Verification items for the finished model (mm, model axes). Face numbers are marked on the shaded views. A direction names the side the tool comes from. Coordinates: 2 decimals unless noted, no trailing zeros. Loops run counter-clockwise (first coordinate to the right, second up) from the corner with the lowest first, then second, coordinate; pieces in that order, holes last. Notation, with made-up numbers: (23, 63) -> (37, 63) arc R29 ccw to (37, 97) -> close; hole circle Ø9 at (79, 41.25). An arc over 180 degrees is marked (long way). Write item = value, one per line.
Autodesk Inventor part; units mm, degrees
ref_plane "Work Plane2" through (-20, 0, -10) normal (0, 0, 1) x (1, 0, 0)
ref_plane "Work Plane3" through (0, 8, 0) normal (0, 1, 0) x (1, 0, 0)
ref_plane "YZ Plane" through (0, 0, 0) normal (1, 0, 0) x (0, 1, 0)
sketch "Sketch1" plane through (0, 0, 0) normal (0, 1, 0) x (-1, 0, 0)
  line L0 (0, 0) -> (20, 0)
  line L1 (20, 0) -> (20, -20)
  line L2 (20, -20) -> (0, -20)
  line L3 (0, -20) -> (0, 0)
  dimension "d0" = 20
  dimension "d1" = 20
extrude "Extrusion1" add sketch "Sketch1" along normal blind 10
sketch "Sketch4" plane through (0, 10, 0) normal (0, 1, 0) x (1, 0, 0)
  line L0 (0, 20) -> (-20, 20)
  line L1 (-20, 20) -> (-20, 0)
  line L2 (-20, 0) -> (0, 0)
  line L3 (0, 0) -> (0, 20)
  line L4 (0, 20) -> (-20, 20)
  line L5 (-20, 20) -> (0, 0)
  line L6 (-10.1768, 10.1768) -> (-7.7019, 12.6517)
  line L7 (-7.7019, 12.6517) -> (-5.227, 10.1768)
  line L8 (-5.227, 10.1768) -> (-7.7019, 7.7019)
  line L9 (-7.7019, 7.7019) -> (-10.1768, 10.1768)
  line L10 (-10.1768, 10.1768) -> (-12.6517, 7.7019)
  line L11 (-12.6517, 7.7019) -> (-15.1265, 10.1768)
  line L12 (-15.1265, 10.1768) -> (-12.6517, 12.6517)
  line L13 (-12.6517, 12.6517) -> (-10.1768, 10.1768)
  line L14 (-12.6517, 12.6517) -> (-10.1768, 15.1265)
  line L15 (-10.1768, 15.1265) -> (-7.7019, 12.6517)
  line L16 (-7.7019, 12.6517) -> (-10.1768, 10.1768)
  line L17 (-10.1768, 10.1768) -> (-12.6517, 12.6517)
  line L18 (-12.6517, 7.7019) -> (-10.1768, 10.1768)
  line L19 (-10.1768, 10.1768) -> (-7.7019, 7.7019)
  line L20 (-7.7019, 7.7019) -> (-10.1768, 5.227)
  line L21 (-10.1768, 5.227) -> (-12.6517, 7.7019)
  dimension "d10" = 3.5
  dimension "d11" = 3.5
  dimension "d12" = 3.5
  dimension "d13" = 3.5
extrude "Extrusion3" cut sketch "Sketch4" against normal blind 8 contours L14 L15 L6 L5 | L5 L10 L11 L12 | L20 L21 L10 L5 | L5 L6 L7 L8
sketch "Sketch5" plane through (0, 10, 0) normal (0, 1, 0) x (1, 0, 0)
  line L0 (-5.227, 10.1768) -> (-10.1768, 5.227)
  line L1 (-10.1768, 5.227) -> (-15.1265, 10.1768)
  line L2 (-15.1265, 10.1768) -> (-10.1768, 15.1265)
  line L3 (-10.1768, 15.1265) -> (-5.227, 10.1768)
  line L4 (0, 20) -> (-20, 20)
  line L5 (-20, 20) -> (-20, 0)
  line L6 (-20, 0) -> (0, 0)
  line L7 (0, 0) -> (0, 20)
  line L8 (-18, 18) -> (-2, 18)
  line L9 (-2, 18) -> (-2, 2)
  line L10 (-2, 2) -> (-18, 2)
  line L11 (-18, 2) -> (-18, 18)
  line L12 (-18, 2) -> (-18, 0)
  line L13 (-2, 2) -> (-2, 0)
  line L14 (-20, 0) -> (0, 0)
  line L15 (-18, 2) -> (-20, 2)
  line L16 (-20, 20) -> (-20, 0)
  line L17 (-2, 2) -> (0, 2)
  line L18 (0, 0) -> (0, 20)
  point P0 (0, 2)
  dimension "d16" = 2
extrude "Extrusion4" add sketch "Sketch5" along normal blind 27 contours L7 L17 L9 L8 L11 L15 L5 L4
ref_plane "Work Plane1" through (-10, 10, -2) normal (1, 0, 0) x (0, 0, -1)
sketch "Sketch6" plane through (-10, 10, -2) normal (1, 0, 0) x (0, 0, -1)
  line L0 (3.227, 0) -> (8.1768, 0)
  line L1 (3.227, 0) -> (3.227, -8)
  line L2 (3.227, -8) -> (8.1768, -8)
  line L3 (8.1768, 0) -> (8.1768, -8)
  line L4 (8.1768, 0) -> (13.1265, 0)
  line L5 (8.1768, 0) -> (8.1768, -8)
  line L6 (8.1768, -8) -> (13.1265, -8)
  line L7 (13.1265, 0) -> (13.1265, -8)
  line L8 (16, 0) -> (0, 0)
  line L9 (16, 0) -> (16, 27)
  line L10 (0, 27) -> (16, 27)
  line L11 (0, 0) -> (0, 27)
  line L12 (8.1768, 0) -> (8.1768, -8)
  line L13 (8.1768, -8) -> (8.1768, -7.25)
  circle A0 centre (8.1768, -7.25) radius 0.75
  point P0 (-2, -10)
  dimension "d20" = 0.75
  dimension "d21" = 1.5
extrude "Extrusion5" cut sketch "Sketch6" along normal mid plane 27 contours A0 L3 | L3 A0
ref_plane "Work Plane2" through (-20, 0, -10) normal (0, 0, 1) x (1, 0, 0)
sketch "Sketch8" plane through (-20, 10, -2) normal (0, 0, 1) x (1, 0, 0)
  line L0 (2, 0) -> (0, 0)
  line L1 (2, 0) -> (2, 27)
  line L2 (0, 27) -> (2, 27)
  line L3 (0, 0) -> (0, 27)
  line L4 (20, 0) -> (18, 0)
  line L5 (20, 0) -> (20, 27)
  line L6 (18, 27) -> (20, 27)
  line L7 (18, 0) -> (18, 27)
  line L8 (20, 27) -> (0, 27)
  line L9 (0, 27) -> (20, 27)
  line L10 (20, 27) -> (20, 25)
  line L11 (20, 25) -> (0, 25)
  line L12 (0, 25) -> (0, 27)
  point P0 (20, -10)
  point P1 (0, 25)
  dimension "d30" = 20
  dimension "d31" = 2
extrude "Extrusion6" add sketch "Sketch8" along normal blind 2 contours L11 L3 L2 L1 | L1 L8 L7 L11 | L7 L6 L5 L11
ref_plane "Work Plane3" through (0, 8, 0) normal (0, 1, 0) x (1, 0, 0)
sketch "Sketch9" plane through (0, 8, 0) normal (0, 1, 0) x (1, 0, 0)
  line L0 (-10.1768, 15.1265) -> (-5.227, 10.1768)
  line L1 (-15.1265, 10.1768) -> (-10.1768, 15.1265)
  line L2 (-10.1768, 5.227) -> (-15.1265, 10.1768)
  line L3 (-5.227, 10.1768) -> (-10.1768, 5.227)
  line L4 (-6.6412, 10.1768) -> (-10.1768, 13.7123)
  line L5 (-10.1768, 13.7123) -> (-13.7123, 10.1768)
  line L6 (-13.7123, 10.1768) -> (-10.1768, 6.6412)
  line L7 (-10.1768, 6.6412) -> (-6.6412, 10.1768)
  point P0 (0, 0)
  dimension "d35" = 1
extrude "Extrusion7" add sketch "Sketch9" against normal blind 6
extrude "Extrusion8" cut sketch "Sketch6" along normal mid plane 27 contours A0 L3 | L3 A0
sketch "Sketch10" plane through (0, 0, 0) normal (1, 0, 0) x (0, 0, -1)
  line L0 (0, 0) -> (20, 0)
  line L1 (20, 0) -> (20, 37)
  line L2 (20, 37) -> (0, 37)
  line L3 (0, 35) -> (0, 37)
  line L4 (2, 35) -> (0, 35)
  line L5 (2, 10) -> (2, 35)
  line L6 (0, 10) -> (2, 10)
  line L7 (0, 0) -> (0, 10)
  line L8 (2, 35) -> (10, 35)
  line L9 (10, 35) -> (4.5, 35)
  line L10 (4.5, 35) -> (4.5, 30)
  line L11 (4.5, 30) -> (17, 30)
  line L12 (17, 30) -> (17, 17.5)
  line L13 (17, 17.5) -> (4.5, 17.5)
  line L14 (4.5, 17.5) -> (4.5, 30)
  dimension "d40" = 5.5
  dimension "d41" = 5
  dimension "d42" = 12.5
  dimension "d43" = 12.5
  dimension "d44" = 8
extrude "Extrusion9" cut sketch "Sketch10" against normal blind 6 contours L11 L12 L13 L14
move faces "Move1" translate (0, -3, 0) faces at (-8.5269, 8, -13.0052)
move faces "Move3" translate (0, -3, 0) faces at (-5.8013, 10, -5.8013)
sketch "Sketch12" plane through (-10, 10, -2) normal (1, 0, 0) x (0, 0, -1)
  circle A0 centre (8, -7.25) radius 0.75
  point P0 (-2, -10)
extrude "Extrusion10" cut sketch "Sketch12" along normal mid plane 100
sketch "Sketch13" plane through (0, 0, 0) normal (1, 0, 0) x (0, 0, -1)
  arc A0 (10.0884, 3.4948) -> (10, 2) centre (10, 2.75) ccw
  circle A1 centre (10, 2.75) radius 1.25
  point P0 (0, 0)
  dimension "d58" = 2.5
extrude "Extrusion11" cut sketch "Sketch13" along normal mid plane 500
properties part number "latticeChamberv6"
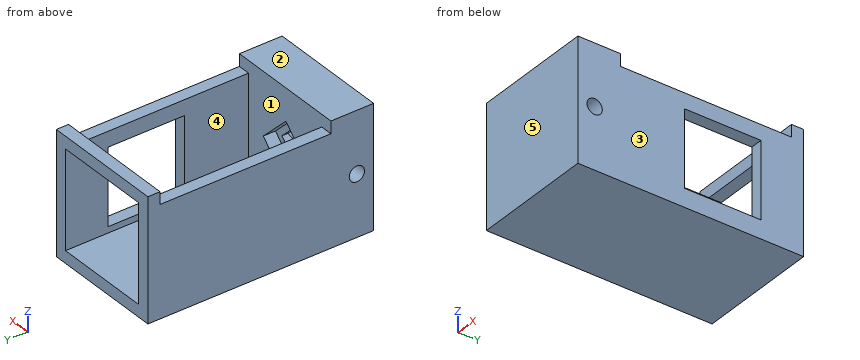
1) Release check for a two-part mould opening along X. For the marked faces 1, 2 and 3 record: pulls with the +X half, pulls with the -X half, needs draft (parallel to the pull), parting line crosses it, or undercut.
Ans:
face_1 = undercut
face_2 = needs draft
face_3 = pulls with the +X half
2) Tool access check on the marked faces 4 and 5. Record the directions out of +Z, -Z, +X, -X, +Y, -Y that give a thin tool (end or side, any length) a straight path to the whole face; none if there is none.
Ans:
face_4 = +Y
face_5 = +Z, -Z, +X, -X, -Y
3) Sectioned sample at C-C, the plane x = -18.5. Record the cut outline in (y, z), plus the area to 3 significant figures.
Ans:
outline = (0, -20) -> (37, -20) -> (37, 0) -> (35, 0) -> (35, -2) -> (7, -2) -> (7, 0) -> (0, 0) -> close; hole circle Ø2.5 at (2.75, -10)
area = 679 mm2
4) Material ranges on line 1 (X direction, y = 9, z = -5.75); line 2 (Z direction, x = -14.25, y = 2.75); line 3 (Y direction, x = -2.25, z = -1.25), recorded low to high.
Ans:
line_1 = -20 to -18, -2 to 0
line_2 = -20 to -11.25, -8.75 to 0
line_3 = 0 to 7, 35 to 37
5) Sectioned sample at B-B, the plane y = 18. Record the cut outline in (x, z).
Ans:
outline = (-20, -20) -> (0, -20) -> (0, -17) -> (-2, -17) -> (-2, -18) -> (-18, -18) -> (-18, -2) -> (-20, -2) -> close; (-2, -4.5) -> (0, -4.5) -> (0, -2) -> (-2, -2) -> close
6) Sectioned sample at A-A, the plane x = -15.5. Record the cut outline in (y, z), plus the area to 3 significant figures.
Ans:
outline = (0, -20) -> (37, -20) -> (37, -18) -> (7, -18) -> (7, 0) -> (0, 0) -> close; (35, -2) -> (37, -2) -> (37, 0) -> (35, 0) -> close; hole circle Ø2.5 at (2.75, -10)
area = 199 mm2
7) Sectioned sample at D-D, the plane z = -6.25. Record the cut outline in (x, y).
Ans:
outline = (-20, 0) -> (0, 0) -> (0, 17.5) -> (-2, 17.5) -> (-2, 7) -> (-9.15, 7) -> (-9.15, 5) -> (-11.2, 5) -> (-11.2, 7) -> (-18, 7) -> (-18, 37) -> (-20, 37) -> close; (-2, 30) -> (0, 30) -> (0, 37) -> (-2, 37) -> close
8) Depth check by flat-ended pin: pin 1 Ø1 at (x, z) = (-12, -1) entering from -Y; pin 2 Ø6 at (x, z) = (-13, -9.5) entering from +Y; pin 3 Ø1 at (x, y) = (-1, 24) entering from +Z; pin 4 Ø1.4 at (x, z) = (-9, -12) entering from +Y. Enter the tip coordinate at first touch or a pass-through.
Ans:
pin_1 = 0
pin_2 = 7
pin_3 = -2
pin_4 = 5
